Input: dimensioned drawing with shaded views. Units: mm. Origin: part minimum x, y, z. A direction names the side the tool comes from. Coordinates: 2 decimals unless noted, no trailing zeros. Loops run counter-clockwise (first coordinate to the right, second up) from the corner with the lowest first, then second, coordinate; pieces in that order, holes last.
Item 1: Section query D-D, the plane y = 6.75. Return the cut outline in (x, z).
Item 2: Section query C-C, the plane x = 59.69. Return the cut outline in (y, z).
Item 3: Pin query (flat end, axial travel): pin 1 Ø6.5 at (y, z) = (6, 91) entering from +X; pin 2 Ø5 at (x, y) = (88.5, 13) entering from +Z; pin 3 Ø3 at (x, z) = (48.5, 101.5) entering from -Y; pin 4 Ø5 at (x, y) = (169.5, 10.5) entering from +Z. Return the tip coordinate at first contact, or that it passes through.
Item 4: Section query B-B, the plane x = 165.1. Return the cut outline in (y, z).
Item 5: Reachability of the marked faces 1 and 2 from +Z, -Z, +X, -X, +Y, -Y: full face, straight path, thin tool, end or side. Return the list, or none.
Item 6: Section query A-A, the plane z = 30.48. Return the cut outline in (x, y).
Item 7: Line query: probe 1 along Y at (x, z) = (118, 124); probe 2 along X at (y, z) = (1.55, 30.48); probe 3 along Z at (x, y) = (101, 7). Output: solid intervals per line, ascending.
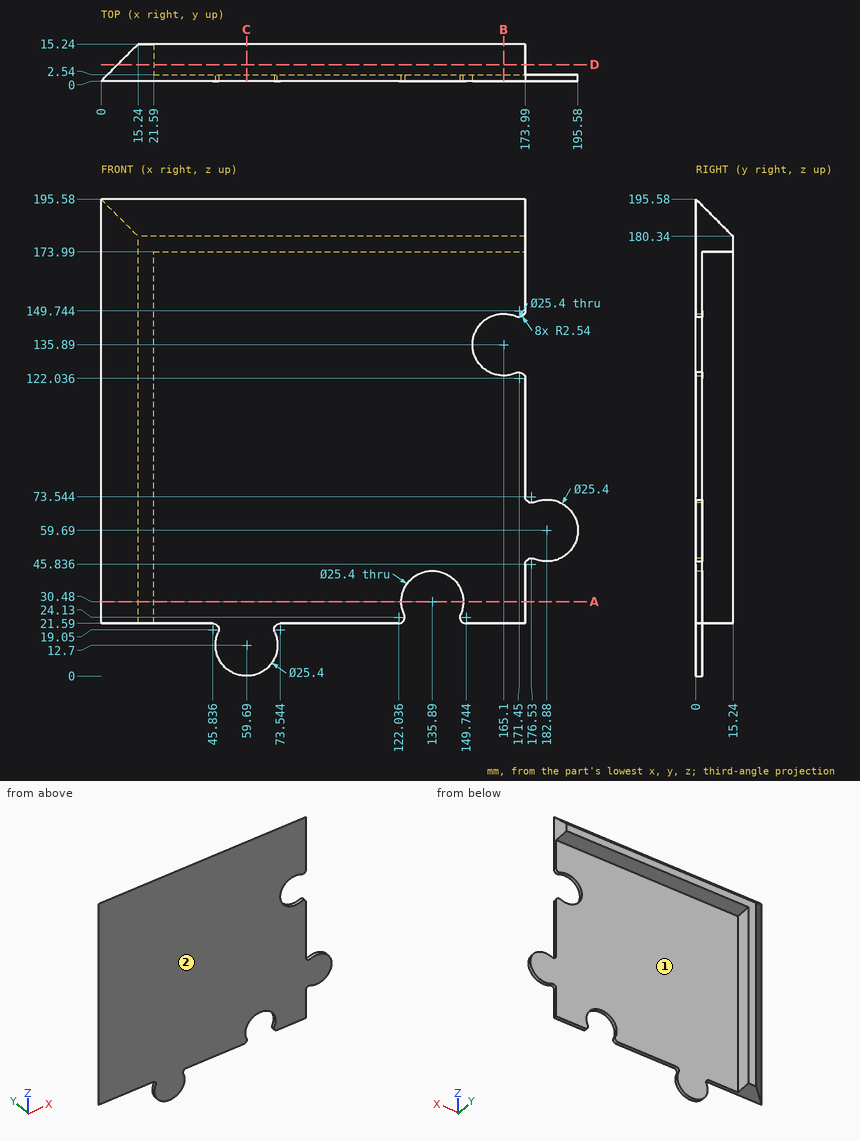
Verdict:
1. outline: (6.75, 21.59) - (21.59, 21.59) - (21.59, 173.99) - (173.99, 173.99) - (173.99, 188.83) - (6.75, 188.83) - close
2. outline: (0, 0) - (2.54, 0) - (2.54, 173.99) - (15.24, 173.99) - (15.24, 180.34) - (0, 195.58) - close
3. pin 1: stops at x = 21.59
3. pin 2: stops at z = 185.08
3. pin 3: stops at y = 0
3. pin 4: stops at z = 187.58
4. outline: (0, 21.59) - (2.54, 21.59) - (2.54, 123.19) - (0, 123.19) - close; (0, 148.59) - (2.54, 148.59) - (2.54, 173.99) - (15.24, 173.99) - (15.24, 180.34) - (0, 195.58) - close
5. face 1: -Z, +X, +Y
5. face 2: +Z, -Z, +X, -X, -Y
6. outline: (0, 0) - (123.19, 0) - (123.19, 2.54) - (21.59, 2.54) - (21.59, 15.24) - (15.24, 15.24) - close; (148.59, 0) - (173.99, 0) - (173.99, 2.54) - (148.59, 2.54) - close
7. probe 1: y = 0 to 2.54
7. probe 2: x = 1.55 to 123.19, 148.59 to 173.99
7. probe 3: z = 173.99 to 188.58
